```python
from build123d import *

# Parameters (mm, degrees)
EXTRUDE_THIN1_DEPTH     = 60
BOSS_EXTRUDE1_DEPTH     = 16
CUT_EXTRUDE1_DEPTH      = 105.764405022
CUT_EXTRUDE2_DEPTH      = 112.059105885
FILLET2_R               = 2
CUT_EXTRUDE3_DEPTH      = 112.059105885
CUT_EXTRUDE3_DEPTH_BACK = 112.059105885
SKETCH6_R               = 2.6
CUT_EXTRUDE4_DEPTH      = 105.764405022
CUT_EXTRUDE4_DEPTH_BACK = 105.764405022
SKETCH7_W               = 78.423709943
SKETCH7_H               = 52.802383793
SKETCH8_W               = 51.319796382
SKETCH8_H               = 40.051163843
BOSS_EXTRUDE2_DEPTH     = 16
SKETCH9_W               = 91.777168916
SKETCH9_H               = 33.81264118
CUT_EXTRUDE5_DEPTH      = 95.816269701
SKETCH12_W              = 62.932503526
SKETCH12_H              = 35
SKETCH12_R              = 4
BOSS_EXTRUDE5_DEPTH     = 11
CUT_EXTRUDE6_DEPTH      = 96.368364776
CUT_EXTRUDE6_DEPTH_BACK = 96.368364776
SKETCH13_W              = 157.086871367
SKETCH13_H              = 169.783274599
SKETCH13_W_2            = 59.932503526
SKETCH13_H_2            = 122.233999749
FILLET6_R               = 6
SKETCH14_R              = 1.75
CUT_EXTRUDE7_DEPTH      = 15
CUT_EXTRUDE8_DEPTH      = 30


with BuildPart() as part:
    # Sketch1 → Extrude-Thin1 (new body)
    with BuildSketch(Plane(origin=(0, 0, 0), x_dir=(1, 0, 0), z_dir=(0, 1, 0))):
        Polygon((-28.637824638, -0.353553391), (0, -28.991378029), (28.637824638, -0.353553391), (31.466251763, -3.181980515), (0, -34.648232278), (-31.466251763, -3.181980515), align=None)
    extrude(amount=EXTRUDE_THIN1_DEPTH)

    # Sketch2 → Boss-Extrude1 (add)
    with BuildSketch(Plane(origin=(0, 0, 0), x_dir=(1, 0, 0), z_dir=(0, 1, 0))):
        with BuildLine():
            Line((-31.466251763, -3.181980515), (-31.466251763, -88))
            Line((-31.466251763, -88), (-2, -88))
            Line((-2, -88), (-2, -69.17683529))
            ThreePointArc((-2, -69.17683529), (0, -36.7), (2, -69.17683529))
            Line((2, -69.17683529), (2, -88))
            Line((2, -88), (31.466251763, -88))
            Line((31.466251763, -88), (31.466251763, -3.181980515))
            Line((31.466251763, -3.181980515), (0, -34.648232278))
            Line((0, -34.648232278), (-31.466251763, -3.181980515))
        make_face()
    extrude(amount=BOSS_EXTRUDE1_DEPTH)

    # Sketch3 → Cut-Extrude1 (cut, through all)
    with BuildSketch(Plane(origin=(17.324116139, 0, 17.324116139), x_dir=(0.7071067811865475, 0, -0.7071067811865476), z_dir=(0.7071067811865476, 0, 0.7071067811865475))):
        with BuildLine():
            Line((2.75, 50), (2.75, 20))
            ThreePointArc((2.75, 20), (0, 17.25), (-2.75, 20))
            Line((-2.75, 20), (-2.75, 50))
            ThreePointArc((-2.75, 50), (0, 52.75), (2.75, 50))
        make_face()
    cut_extrude1 = extrude(amount=-CUT_EXTRUDE1_DEPTH, mode=Mode.SUBTRACT)

    # Mirror1: Cut-Extrude1 across plane
    add(cut_extrude1.mirror(Plane(origin=(0, 0, 0), x_dir=(0, 0, 1), z_dir=(1, 0, 0))), mode=Mode.SUBTRACT)

    # Sketch5 → Cut-Extrude2 (cut, through all)
    with BuildSketch(Plane(origin=(0, 0, 0), x_dir=(1, 0, 0), z_dir=(0, 1, 0))):
        with BuildLine():
            Line((-31.466251763, -21.533748237), (-17.182694783, -35.817305217))
            ThreePointArc((-17.182694783, -35.817305217), (-23.904625503, -57.365647669), (-10, -75.147008827))
            Line((-10, -75.147008827), (-10, -88))
            Line((-10, -88), (-31.466251763, -88))
            Line((-31.466251763, -88), (-31.466251763, -21.533748237))
        make_face()
    cut_extrude2 = extrude(amount=CUT_EXTRUDE2_DEPTH, mode=Mode.SUBTRACT)

    # Mirror2: Cut-Extrude2 across plane
    add(cut_extrude2.mirror(Plane(origin=(0, 0, 0), x_dir=(0, 0, 1), z_dir=(1, 0, 0))), mode=Mode.SUBTRACT)

    # Fillet2
    fillet2_edges = [part.edges().sort_by_distance(p)[0] for p in [
        (10, 8, 75.147008827),
        (-10, 8, 75.147008827),
    ]]
    fillet(fillet2_edges, radius=FILLET2_R)

    # Sketch6 → Cut-Extrude3 (cut, two sides: drawn at the far end of the back side and taken through both)
    with BuildSketch(Plane(origin=(0, 0, 0), x_dir=(0, 0, -1), z_dir=(1, 0, 0)).offset(-CUT_EXTRUDE3_DEPTH_BACK)):
        with Locations((-82, 8)):
            Circle(SKETCH6_R)
    extrude(amount=CUT_EXTRUDE3_DEPTH + CUT_EXTRUDE3_DEPTH_BACK, mode=Mode.SUBTRACT)

    # Sketch7 → Cut-Extrude4 (cut, two sides: drawn at the far end of the back side and taken through both)
    with BuildSketch(Plane(origin=(-17.324116139, 0, 17.324116139), x_dir=(0.7071067811865475, 0, 0.7071067811865476), z_dir=(-0.7071067811865476, 0, 0.7071067811865475)).offset(-CUT_EXTRUDE4_DEPTH_BACK)):
        with Locations((-0.892385334, 42.401191897)):
            Rectangle(SKETCH7_W, SKETCH7_H)
    extrude(amount=CUT_EXTRUDE4_DEPTH + CUT_EXTRUDE4_DEPTH_BACK, mode=Mode.SUBTRACT)

    # Sketch8 → Boss-Extrude2 (add)
    with BuildSketch(Plane(origin=(0, 16, 0), x_dir=(1, 0, 0), z_dir=(0, 1, 0))):
        with Locations((0.329762311, -10.635090251)):
            Rectangle(SKETCH8_W, SKETCH8_H)
    extrude(amount=-BOSS_EXTRUDE2_DEPTH)

    # Sketch9 → Cut-Extrude5 (cut, through all)
    with BuildSketch(Plane(origin=(0, 16, 0), x_dir=(1, 0, 0), z_dir=(0, 1, 0))):
        with Locations((0.452847873, -5.06743142)):
            Rectangle(SKETCH9_W, SKETCH9_H)
    extrude(amount=-CUT_EXTRUDE5_DEPTH, mode=Mode.SUBTRACT)

    # Sketch12 → Boss-Extrude5 (add)
    with BuildSketch(Plane(origin=(0, 0, 21.97375201), x_dir=(-1, 0, 0), z_dir=(0, 0, -1))):
        with Locations((0, 17.5)):
            Rectangle(SKETCH12_W, SKETCH12_H)
        with Locations((-15, 25)):
            Circle(SKETCH12_R, mode=Mode.SUBTRACT)
        with Locations((15, 25)):
            Circle(SKETCH12_R, mode=Mode.SUBTRACT)
    extrude(amount=BOSS_EXTRUDE5_DEPTH)

    # Sketch13 → Cut-Extrude6 (cut, two sides: drawn at the far end of the back side and taken through both)
    with BuildSketch(Plane(origin=(0, 16, 0), x_dir=(1, 0, 0), z_dir=(0, 1, 0)).offset(-CUT_EXTRUDE6_DEPTH_BACK)):
        with Locations((-2.365016289, -53.735825088)):
            Rectangle(SKETCH13_W, SKETCH13_H)
        with Locations((0, -51.3708088)):
            Rectangle(SKETCH13_W_2, SKETCH13_H_2, mode=Mode.SUBTRACT)
    extrude(amount=CUT_EXTRUDE6_DEPTH + CUT_EXTRUDE6_DEPTH_BACK, mode=Mode.SUBTRACT)

    # Fillet6
    fillet6_edges = [part.edges().sort_by_distance(p)[0] for p in [
        (17.182694783, 8, 35.817305217),
        (-17.182694783, 8, 35.817305217),
    ]]
    fillet(fillet6_edges, radius=FILLET6_R)

    # Sketch14 → Cut-Extrude7 (cut)
    with BuildSketch(Plane(origin=(0, 0, 10.97375201), x_dir=(-1, 0, 0), z_dir=(0, 0, -1))):
        with Locations((0, 10)):
            Circle(SKETCH14_R)
    extrude(amount=-CUT_EXTRUDE7_DEPTH, mode=Mode.SUBTRACT)

    # Sketch15 → Cut-Extrude8 (cut)
    with BuildSketch(Plane(origin=(0, 16, 0), x_dir=(1, 0, 0), z_dir=(0, 1, 0))):
        Polygon((25.989660502, -27.010339498), (22.339327827, -30.660672173), (25.989660502, -30.660672173), align=None)
        Polygon((-25.989660502, -30.660672173), (-25.989660502, -27.010339498), (-22.339327827, -30.660672173), align=None)
    extrude(amount=-CUT_EXTRUDE8_DEPTH, mode=Mode.SUBTRACT)


solid = part.part
```
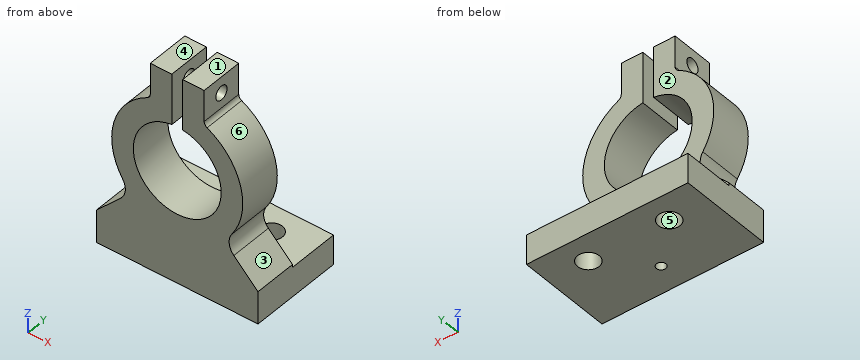
Check sheet for the modelled part. Datum: model origin and axes. Units: mm. Face numbers are marked on the shaded views. A direction names the side the tool comes from. Coordinates: 2 decimals unless noted, no trailing zeros. Write each loop counter-clockwise with the first axis right and the second up, starting at its lowest first coordinate (ties: lowest second). Pieces come first, ordered by that corner, then holes. Notation, with made-up numbers: M 23,27 L 69,27 A15 ccw 69,43 Z; hole C 18.25,-33 d2. An arc over 180 degrees is marked long. Write item = value, one per line. Start each with the question number.
1. Sectioned sample at D-D (x = 13). Record the cut outline in (y, z).
2. Tool access check on the marked faces 1, 2 and 3. Record the directions out of +Z, -Z, +X, -X, +Y, -Y that give a thin tool (end or side, any length) a straight path to the whole face; none if there is none.
3. Go/stop test with flat-tipped pins: pin 1 (21 mm diameter, centred on x = 14, y = 29.5, fed in from +Z); pin 2 (9.5 mm diameter, centred on y = 5.5, z = 85, fed in from -X); pin 3 (7 mm diameter, centred on y = 8, z = 82, fed in from +X); pin 4 (4 mm diameter, centred on x = 0, y = 10, fed in from -Z). Record where each tip stops, or that it passes through.
4. Mould release check, pull along Z, two halves, no side actions. Record for the marked faces 4, 5 and 6: pulls with the +Z half, pulls with the -Z half, needs draft (parallel to the pull), parting line crosses it, or undercut.
5. Thickness scan on probe 1 along Y at (x, z) = (-8, 82); probe 2 along Y at (x, z) = (-15, 15); probe 3 along Z at (x, y) = (4, 10). Record the ranges inside material, lowest first.
6. Sectioned sample at A-A (x = 7). Record the cut outline in (y, z), then the cut area to 3 significant figures.
7. Sectioned sample at C-C (y = 22). Record the cut outline in (x, z).
8. Sectioned sample at B-B (z = 53). Record the cut outline in (x, y), then the cut area to 3 significant figures.
The answers:
q1.outline = M 0,10.97 L 21.54,10.97 L 21.54,21.97 L 16,21.97 L 16,43.17 L 0,43.17 Z; M 0,62.83 L 16,62.83 L 16,73.53 L 0,73.53 Z; M 28.46,10.97 L 35,10.97 L 35,21.97 L 28.46,21.97 Z
q2.face_1 = +Z, +X, -X, +Y, -Y
q2.face_2 = +Z, +X, -X, +Y
q2.face_3 = +X, +Y, -Y
q3.pin_1 = 21.97
q3.pin_2 = -10
q3.pin_3 = 10
q3.pin_4 = 10.97
q4.face_4 = pulls with the +Z half
q4.face_5 = needs draft
q4.face_6 = undercut
q5.probe_1 = 0 to 5.4, 10.6 to 16
q5.probe_2 = 0 to 21, 29 to 35
q5.probe_3 = 10.97 to 37.2, 68.8 to 80.34, 83.66 to 88
q6.outline = M 0,10.97 L 35,10.97 L 35,21.97 L 16,21.97 L 16,38.28 L 0,38.28 Z; M 0,67.72 L 16,67.72 L 16,88 L 0,88 Z; hole C 8,82 d5.2
q6.area = 949 mm²
q7.outline = M -29.97,10.97 L -17.65,10.97 L -17.65,21.97 L -29.97,21.97 Z; M -12.35,10.97 L 12.35,10.97 L 12.35,21.97 L -12.35,21.97 Z; M 17.65,10.97 L 29.97,10.97 L 29.97,21.97 L 17.65,21.97 Z
q8.outline = M -24.3,0 L -16.3,0 L -16.3,16 L -24.3,16 Z; M 16.3,0 L 24.3,0 L 24.3,16 L 16.3,16 Z
q8.area = 256 mm²
